Verification items for this drawing (mm, ordinates from the low corner). A direction names the side the tool comes from. Give positions to 0.01 mm unless a question says otherwise; leave off trailing zeros. Order: outer loops, then holes, each group sorted by start corner. A loop starts at its lowest first (then second) coordinate and runs counter-clockwise, first axis right, second up.
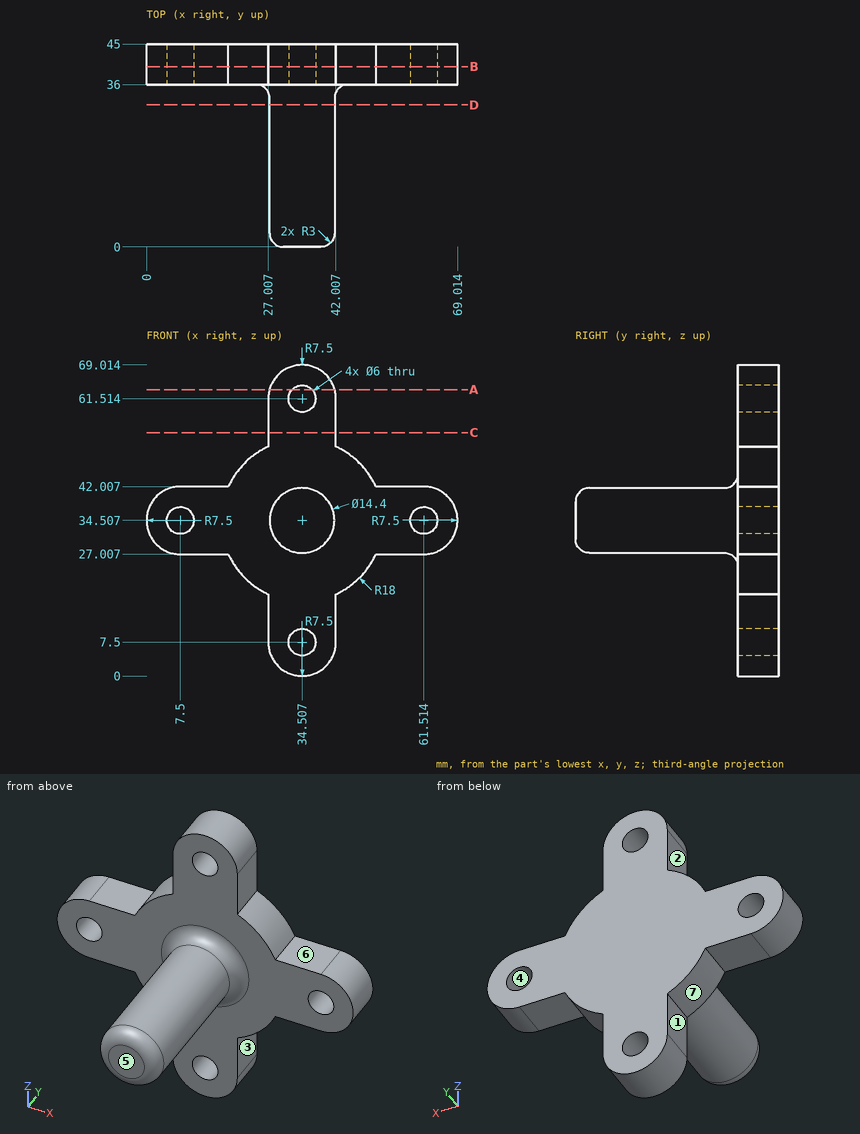
Q1. Cross-section at B-B, the plane y = 40. Record the boundary of the cut face in (x, z), and give its area (3 significant figures).
Q2. Release check for a two-part mould opening along Z. For the marked faces 4, 5, 6 and 7 record: pulls with the +Z half, pulls with the -Z half, needs draft (parallel to the pull), parting line crosses it, or undercut.
Q3. Cross-section at C-C, the plane z = 54. Record the boundary of the cut face in (x, y).
Q4. Thickness scan on L1, parallel to Y at x = 53.5, z = 33.5; L2, parallel to X at y = 36.5, z = 12. Record the ranges inside material, lowest first.
Q5. Cross-section at D-D, the plane y = 31.5. Record the boundary of the cut face in (x, z).
Q6. Access from +Z, -Z, +X, -X, +Y, -Y to the whole of each face (thin tool, end or side, straight path). Record for the marked faces 1, 2 and 3.
Q7. Cross-section at A-A, the plane z = 63.5. Record the boundary of the cut face in (x, y) (1 decimal).
Q8. Gauge pin test, flat ends, axial feed: P1, Ø8, axis at x = 40, y = 15, coming from the +Z side; P2, Ø3.5, axis at x = 34.51, z = 7.5, coming from the -Y side; P3, Ø10, axis at x = 34, z = 60, coming from the -Y side; P4, Ø7, axis at x = 57, y = 42, coming from the +Z side. Record the tip position at first contact, or that the pin passes through.
Answers follow:
1. outline: (7.5, 27.01) - (18.14, 27.01) arc R18 ccw to (27.01, 18.14) - (27.01, 7.51) arc R7.5 ccw to (42.01, 7.5) - (42.01, 18.14) arc R18 ccw to (50.87, 27.01) - (61.51, 27.01) arc R7.5 ccw to (61.51, 42.01) - (50.87, 42.01) arc R18 ccw to (42.01, 50.87) - (42.01, 61.51) arc R7.5 ccw to (27.01, 61.51) - (27.01, 50.87) arc R18 ccw to (18.14, 42.01) - (7.51, 42.01) arc R7.5 ccw to start; hole circle Ø6 at (7.5, 34.51); hole circle Ø6 at (34.51, 7.5); hole circle Ø6 at (34.51, 61.51); hole circle Ø6 at (61.51, 34.51)
1. area: 1,830 mm2
2. face 4: undercut
2. face 5: needs draft
2. face 6: pulls with the +Z half
2. face 7: pulls with the -Z half
3. outline: (27.01, 36) - (42.01, 36) - (42.01, 45) - (27.01, 45) - close
4. L1: y = 36 to 45
4. L2: x = 27.01 to 42.01
5. outline: circle Ø14.4 at (34.51, 34.51)
6. face 1: -Z, -X, +Y, -Y
6. face 2: +Z, -X, +Y, -Y
6. face 3: -Z, +X, +Y, -Y
7. outline: (27.3, 36) - (32.3, 36) - (32.3, 45) - (27.3, 45) - close; (36.8, 36) - (41.7, 36) - (41.7, 45) - (36.8, 45) - close
8. P1: stops at z = 41.55
8. P2: passes through
8. P3: stops at y = 36
8. P4: stops at z = 42.01
